The model under review builds one solid part; all positions refer to its coordinate system, in mm. Face numbers are marked on the shaded views. Give positions to 0.01 mm unless a question says otherwise; leave off trailing zeros. Loops run counter-clockwise (first coordinate to the right, second up) from the corner with the lowest first, then second, coordinate; pieces in that order, holes last. Notation, with made-up numbers: M 31.25,43 L 52.25,43 A13 ccw 52.25,62 Z; hole C 52,36.25 d11. An arc over 180 degrees is marked long. Return JSON: item names as keys, results as strings.
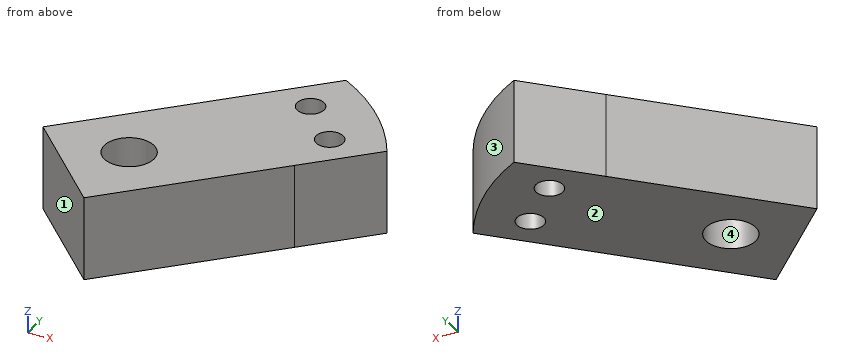
Autodesk Inventor part; units mm, degrees
ref_plane "YZ Plane" through (0, 0, 0) normal (1, 0, 0) x (0, 1, 0)
ref_plane "XZ Plane" through (0, 0, 0) normal (0, 1, 0) x (-1, 0, 0)
ref_plane "XY Plane" through (0, 0, 0) normal (0, 0, 1) x (1, 0, 0)
sketch "Skizze1" plane through (0, 0, 0) normal (0, 0, 1) x (1, 0, 0)
  circle A0 centre (2.5036, -2.4424) radius 1.4 construction
  circle A1 centre (-2.5484, 2.3924) radius 1.4 construction
  arc A2 (8.8953, -1.5488) -> (-1.9335, 8.8203) centre (-14.4319, -15.0709) ccw
  line L0 (-1.9335, 8.8203) -> (-8.8953, 1.5457)
  line L1 (-8.8953, 1.5457) -> (1.9365, -8.8203)
  line L2 (1.9365, -8.8203) -> (8.8953, -1.5488)
  arc A3 (-17.415, -14.7529) -> (-12.7255, -17.5384) centre (-14.4319, -15.0709) ccw
  line L3 (-8.8953, 1.5457) -> (-24.7975, -15.0712)
  line L4 (-24.7975, -15.0712) -> (-13.9657, -25.4371)
  line L5 (-13.9657, -25.4371) -> (1.9365, -8.8203)
  arc A4 (-13.2888, -12.8475) -> (-12.2085, -16.214) centre (-14.4319, -15.0709) ccw
  circle A5 centre (-14.4319, -15.0709) radius 2.95
  circle A6 centre (-2.5484, 2.3924) radius 1.6
  circle A7 centre (2.5036, -2.4424) radius 1.6
  point P0 (0, 0)
  dimension "d0" = 23
  dimension "d1" = 5.9
  dimension "d2" = 3.2
  dimension "d3" = 3.2
extrude "Extrusion1" add sketch "Skizze1" along normal blind 10
sketch "Skizze2" plane through (0, 0, 10) normal (0, 0, 1) x (1, 0, 0)
  point P0 (0, 0)
sketch "Skizze3" plane through (0, 0, 10) normal (0, 0, 1) x (1, 0, 0)
  point P0 (0, 0)
properties part number "IM_Matchboxscope_Laserholder_2"
1) Consider section C-C on z = 1. Write out the cut boundary in (x, y), then the cut area to 3 significant figures.
From the geometry:
{"outline": "M -24.8,-15.07 L -13.97,-25.44 L 1.94,-8.82 L 8.9,-1.55 A26.96 ccw -1.93,8.82 L -8.9,1.55 Z; hole C -14.43,-15.07 d5.9; hole C -2.55,2.39 d3.2; hole C 2.5,-2.44 d3.2", "area": "463 mm²"}
2) Consider section B-B on y = -13.5. Write out the cut boundary in (x, z).
From the geometry:
{"outline": "M -23.29,0 L -16.93,0 L -16.93,10 L -23.29,10 Z; M -11.93,0 L -2.54,0 L -2.54,10 L -11.93,10 Z"}
3) Consider section A-A on x = -2.5. Write out the cut boundary in (y, z), then the cut area to 3 significant figures.
From the geometry:
{"outline": "M -13.46,0 L 0.79,0 L 0.79,10 L -13.46,10 Z; M 3.99,0 L 8.23,0 L 8.23,10 L 3.99,10 Z", "area": "185 mm²"}
4) Consider section D-D on x = -18. Write out the cut boundary in (y, z), then the cut area to 3 significant figures.
From the geometry:
{"outline": "M -21.58,0 L -7.97,0 L -7.97,10 L -21.58,10 Z", "area": "136 mm²"}
5) Wall thickness on L1, parallel to X at y = 2, z = 7.5; L2, parallel to X at y = -1, z = 3.5; L3, parallel to Y at x = -15, z = 2: over which ranges is each line inside the solid? List them lowest first. Write a range as from..to.
From the geometry:
{"L1": "-8.46..-4.1, -1..6.44", "L2": "-11.33..1.81, 3.2..8.57", "L3": "-24.45..-17.97, -12.18..-4.83"}
6) The part is to be moulded in two halves that separate along Y. For the marked faces 1, 2, 3 and 4, say which applies: released by +Y, released by -Y, zero draft, split by the parting line, or undercut.
From the geometry:
{"face 1": "released by -Y", "face 2": "zero draft", "face 3": "released by +Y", "face 4": "undercut"}
7) Insertion check: pin 1 (1.9 mm diameter, centred on x = 2.5, y = -2.44, fed in from +Z); pin 2 (4 mm diameter, centred on x = -9, y = 0, fed in from -Z); pin 3 (1 mm diameter, centred on x = -18.5, z = 2, fed in from -Y); pin 4 (1 mm diameter, centred on x = -14, z = 5.5, fed in from +Y). Each pin has a flat end and moves straight along its axis. Give the tip position at first contact, or say it passes through.
From the geometry:
{"pin 1": "through", "pin 2": "z = 0", "pin 3": "y = -21.58", "pin 4": "y = -3.27"}
